Read the model definition and answer for the solid it produces. Units are mm, in the model's axes. A direction names the side the tool comes from. Coordinates: 2 decimals unless noted, no trailing zeros. Order: outer loops, then holes, each group sorted by start corner. A loop starts at its lowest first (then second) coordinate and runs counter-clockwise, first axis right, second up.
```python
from build123d import *

# Parameters (mm, degrees)
SKETCH2_W             = 10
SKETCH2_H             = 4
EXTRUDE1_DEPTH        = 600
M8_TAPPED_HOLE1_D     = 6.8
M8_TAPPED_HOLE1_DEPTH = 19.75
M8_TAPPED_HOLE1_TIP   = 2.042926105


with BuildPart() as part:
    # Sketch1 → Revolve1 (revolve)
    with BuildSketch(Plane.XY, mode=Mode.PRIVATE) as revolve1_sk:
        Polygon((-108.27123445, 10), (-108.27123445, 0), (491.72876555, 0), (491.72876555, -35.462555066), (501.72876555, -35.462555066), (501.72876555, 10), align=None)
    revolve(revolve1_sk.sketch.rotate(Axis((-148.45814978, 40, 0), (1, 0, 0)), 270), axis=Axis((-148.45814978, 40, 0), (1, 0, 0)))

    # Sketch2 → Extrude1 (cut)
    with BuildSketch(Plane.ZY.offset(108.27123445)):
        with Locations((0, 80)):
            Rectangle(SKETCH2_W, SKETCH2_H)
    extrude(amount=-EXTRUDE1_DEPTH, mode=Mode.SUBTRACT)

    # M8 Tapped Hole1
    with Locations(Plane(origin=(501.72876555, 82.426406871, 42.426406871), x_dir=(0, 0, 1), z_dir=(1, 0, 0))):
        with Locations((0, 0), (-84.852813742, 0), (-84.852813742, 84.852813742), (0, 84.852813742)):
            Hole(M8_TAPPED_HOLE1_D / 2, depth=M8_TAPPED_HOLE1_DEPTH)
            with Locations((0, 0, -(M8_TAPPED_HOLE1_DEPTH + M8_TAPPED_HOLE1_TIP / 2))):  # 118° drill point
                Cone(0, M8_TAPPED_HOLE1_D / 2, M8_TAPPED_HOLE1_TIP, mode=Mode.SUBTRACT)


solid = part.part
```
1) A cutting plane is placed at B-B, the plane x = 310. Determine the outline of the cut face in (y, z), and give its area (3 significant figures).
A:
outline: (78, -5) - (78, 5) - (79.69, 5) arc R40 ccw (long way) to (79.69, -5) - close; hole circle Ø60 at (40, 0)
area: 2,180 mm2
2) A cutting plane is placed at A-A, the plane y = 40. Determine the outline of the cut face in (x, z).
A:
outline: (-108.27, -40) - (491.73, -40) - (491.73, -75.46) - (501.73, -75.46) - (501.73, -30) - (-108.27, -30) - close; (-108.27, 30) - (501.73, 30) - (501.73, 75.46) - (491.73, 75.46) - (491.73, 40) - (-108.27, 40) - close
3) Straight lines are drawn through the part: line 1 (Z direction, x = 387.5, y = 41.5); line 2 (Y direction, x = 286, z = 0); line 3 (X direction, y = -13, z = 5.5). For each, find the intervals that lie inside material, in ascending order.
A:
line 1: z = -39.97 to -29.96, 29.96 to 39.97
line 2: y = 0 to 10, 70 to 78
line 3: x = 491.73 to 501.73
4) A cutting plane is placed at C-C, the plane z = 24. Determine the outline of the cut face in (x, y).
A:
outline: (-108.27, 8) - (491.73, 8) - (491.73, -31.54) - (501.73, -31.54) - (501.73, 22) - (-108.27, 22) - close; (-108.27, 58) - (501.73, 58) - (501.73, 111.54) - (491.73, 111.54) - (491.73, 72) - (-108.27, 72) - close
5) Which of the six approach directions +Z, -Z, +X, -X, +Y, -Y give full straight-line access (tool end or side, diameter ignored) to faces 4 (the flat face through (188, 78, 0)), 5 (the flat face through (-108.271, 10, -6)), 6 (the cylindrical face through (195.929, 0.036, 1.689))?
A:
face 4: -X, +Y
face 5: +Z, -Z, -X, +Y, -Y
face 6: -X
6) A cutting plane is placed at D-D, the plane z = 54.5. Determine the outline of the cut face in (x, y).
A:
outline: (491.73, -12.2) - (501.73, -12.2) - (501.73, 92.2) - (491.73, 92.2) - close
7) Determine the mould class of faces 1 (the flat face through (501.729, 72, -1)), 2 (the cylindrical face through (192.459, 69.287, -6.503)), 3 (the cylindrical face through (496.8, -11, -55.62)) for opening direction Z: pulls with the +Z half, pulls with the -Z half, needs draft (parallel to the pull), parting line crosses it, or undercut.
A:
face 1: needs draft
face 2: undercut
face 3: parting line crosses it
8) Flat-ended cylindrical pins translate along their axes: pin 1 Ø1 at (x, y) = (117.5, 41) entering from +Z; pin 2 Ø10 at (x, z) = (208, 18.5) entering from -Y; pin 3 Ø12 at (y, z) = (-16.5, 3) entering from -X. Find the tip coordinate at first contact, or state that the pin passes through.
A:
pin 1: stops at z = 40
pin 2: stops at y = 2.35
pin 3: stops at x = 491.73
